Verification items for the finished model (mm, model axes). Face numbers are marked on the shaded views. A direction names the side the tool comes from. Coordinates: 2 decimals unless noted, no trailing zeros. Order: outer loops, then holes, each group sorted by start corner. A loop starts at its lowest first (then second) coordinate and runs counter-clockwise, first axis right, second up. Notation, with made-up numbers: M 11,1.25 L 64,1.25 A8 ccw 64,11.25 Z; hole C 82,41.25 d4. An arc over 180 degrees is marked long. Answer as a JSON object with one key per item and string values. Group by question number.
(1) Cross-section at C-C (z = 2.5). Enter the section's corners in (x, y).
(2) Mould release check, pull along Z, two halves, no side actions. Record for the marked faces 1, 2 and 3: released by +Z, released by -Z, zero draft, split by the parting line, or undercut.
(3) Cross-section at D-D (z = 1.5). Enter the section's corners in (x, y).
(4) Access from +Z, -Z, +X, -X, +Y, -Y to the whole of each face (thin tool, end or side, straight path). Record for the marked faces 4 and 5.
(5) Cross-section at B-B (x = 3.5). Enter the section's corners in (y, z), plus the area to 3 significant figures.
(6) Cross-section at A-A (y = 3.45). Enter the section's corners in (x, z).
(7) Gauge pin test, flat end, axial feed: pin 1 Ø2.5 at (x, z) = (4.5, 1.5) entering from +Y. Record the tip position at first contact, or that the pin passes through.
(8) Material ranges on line 1 (X direction, y = 1.45, z = -0.5); line 2 (Z direction, x = 3.5, y = 0.1); line 3 (X direction, y = 2.45, z = 1), recorded low to high.
from build123d import *

# Parameters (mm, degrees)
F0_W          = 12
F0_H          = 6.8
F0_W_2        = 9.6
F0_H_2        = 4.4
F1_DEPTH      = 4
F1_DEPTH_BACK = 2
F3_W          = 0.8
F3_H          = 4
F2_W          = 0.8
F2_H          = 4
F4_DEPTH      = 0.6
F5_W          = 9.6
F5_H          = 4.4
F6_DEPTH      = 2
F7_R          = 1.1
F8_DEPTH      = 12.5


with BuildPart() as f1:
    # F0 (on Front) → F1 (new body, two sides)
    with BuildSketch(Plane.XZ) as f1_sk:
        with Locations((4.8, 2.2)):
            Rectangle(F0_W, F0_H)
        with Locations((4.8, 2.2)):
            Rectangle(F0_W_2, F0_H_2, mode=Mode.SUBTRACT)
    extrude(amount=-F1_DEPTH)
    extrude(f1_sk.sketch, amount=F1_DEPTH_BACK)

    # F3 (on face) + F2 (on face) → F4 (cut)
    with BuildSketch(Plane.XY):
        with Locations((0.4, 2)):
            Rectangle(F3_W, F3_H)
    with BuildSketch(Plane.XY):
        with Locations((9.2, 2)):
            Rectangle(F2_W, F2_H)
    extrude(amount=-F4_DEPTH, mode=Mode.SUBTRACT)

    # F5 (on Front) → F6 (join)
    with BuildSketch(Plane.XZ):
        with Locations((4.8, 2.2)):
            Rectangle(F5_W, F5_H)
    extrude(amount=F6_DEPTH)

    # F7 (on Front) → F8 (cut, symmetric)
    with BuildSketch(Plane.XZ):
        with Locations((1.1, 3.3)):
            Circle(F7_R)
    extrude(amount=F8_DEPTH, both=True, mode=Mode.SUBTRACT)


solid = f1.part
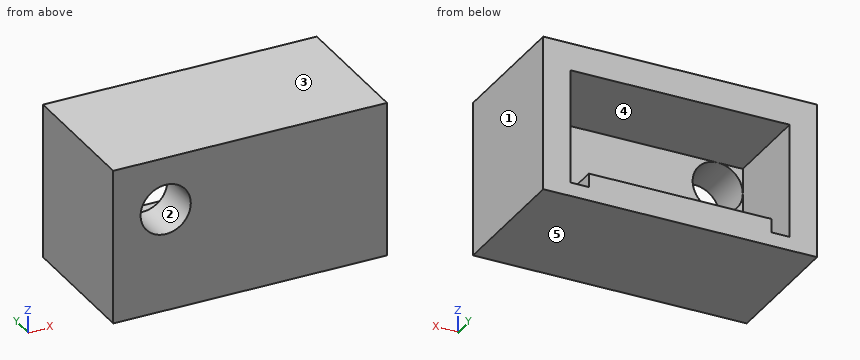
Taken from the geometry:
{
 "1": {"outline": "M -1.2,-2 L 0.35,-2 L 0.35,0 L 0,0 L 0,4 L -1.2,4 Z; M 1.85,-2 L 10.8,-2 L 10.8,4 L 9.6,4 L 9.6,0 L 1.85,0 Z"},
 "2": {"face 1": "zero draft", "face 2": "undercut", "face 3": "released by +Z"},
 "3": {"outline": "M -1.2,-2 L 10.8,-2 L 10.8,4 L 9.6,4 L 9.6,0 L 0,0 L 0,4 L -1.2,4 Z"},
 "4": {"face 4": "+Y", "face 5": "-Z, +X, -X, +Y, -Y"},
 "5": {"outline": "M -2,-1.2 L 4,-1.2 L 4,0 L 0,0 L 0,4.4 L 4,4.4 L 4,5.6 L -2,5.6 Z", "area": "23.2 mm²"},
 "6": {"outline": "M -1.2,-1.2 L 10.8,-1.2 L 10.8,5.6 L -1.2,5.6 Z; hole M 0,-0.6 L 0.8,-0.6 L 0.8,0 L 8.8,0 L 8.8,-0.6 L 9.6,-0.6 L 9.6,4.4 L 0,4.4 Z"},
 "7": {"pin 1": "stops at y = 0"},
 "8": {"line 1": "x = -1.2 to 0, 0.8 to 8.8, 9.6 to 10.8", "line 2": "z = -1.2 to 0, 4.4 to 5.6", "line 3": "x = -1.2 to 0, 9.6 to 10.8"}
}
